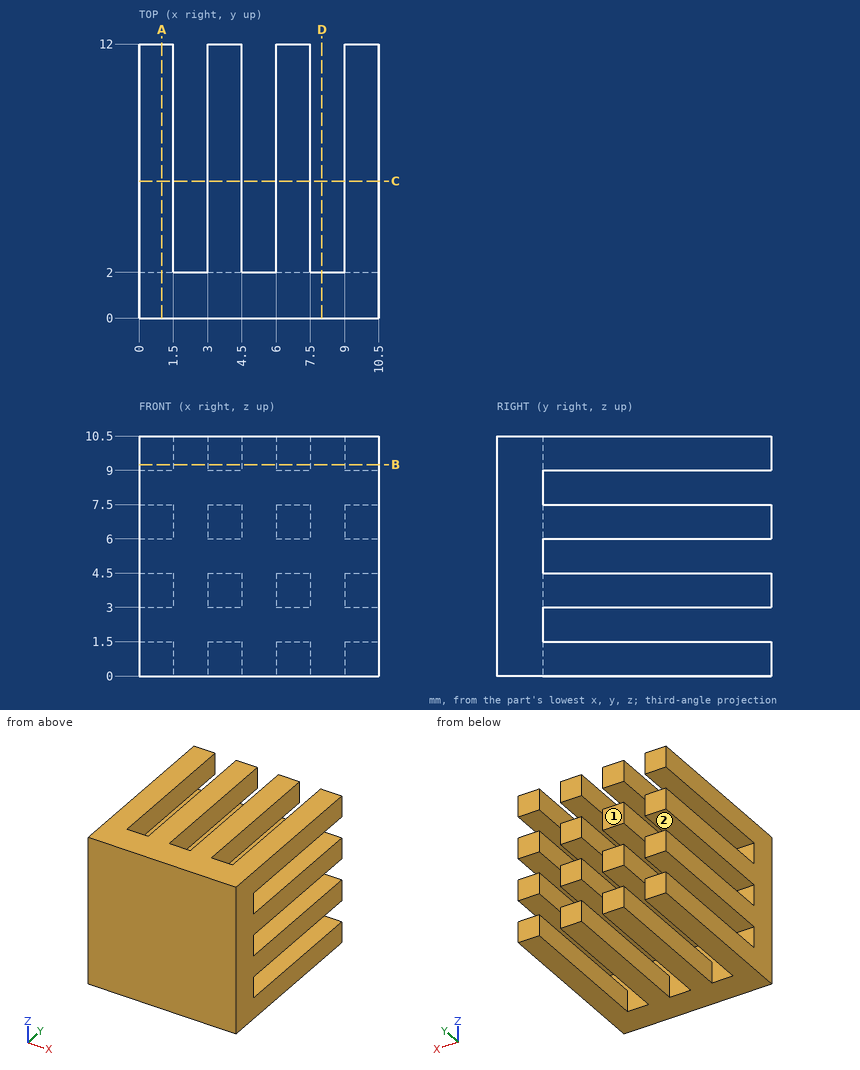
Can you work these out from the drawing? Everything is in mm from the part's minimum corner. A direction names the side the tool comes from. Round coordinates to 2 decimals unless told otherwise and drop trailing zeros. Order: outer loops, then holes, each group sorted by start corner. A loop starts at its lowest first (then second) coordinate and runs counter-clockwise, first axis right, second up. Notation, with made-up numbers: (66.5, 17) -> (109.5, 17) arc R7 ccw to (109.5, 27) -> close; hole circle Ø2 at (28, 60.25). An arc over 180 degrees is marked (long way). Return JSON: item names as keys, results as strings. Group by question number.
1. If we section it at C-C, the plane y = 6: Count the separate pieces of the cut face and the enclosed holes in it, then the cut area to 3 significant figures.
2. I need wall thicknesses on line 1 (Z direction, x = 1.25, y = 4.5); line 2 (Y direction, x = 5.25, z = 2.5). Which ranges of each line are inside material? Lowest first, please. Write a range as [from, to].
3. If we section it at A-A, the plane x = 1: Write out the boundary of the cut face in (y, z), then the cut area to 3 significant figures.
4. If we section it at B-B, the plane z = 9.25: Write out the boundary of the cut face in (x, y), then the cut area to 3 significant figures.
5. Which directions (+Z, -Z, +X, -X, +Y, -Y) give clear straight access to the entire face, cutting with the end or side of a thin tool? Please do the marked faces 1 and 2.
6. If we section it at D-D, the plane x = 8: Write out the boundary of the cut face in (y, z), then the cut area to 3 significant figures.
Output values:
{
 "1": {"separate pieces": "16", "enclosed holes": "0", "area": "36.0 mm²"},
 "2": {"line 1": "[0, 1.5], [3, 4.5], [6, 7.5], [9, 10.5]", "line 2": "[0, 2]"},
 "3": {"outline": "(0, 0) -> (12, 0) -> (12, 1.5) -> (2, 1.5) -> (2, 3) -> (12, 3) -> (12, 4.5) -> (2, 4.5) -> (2, 6) -> (12, 6) -> (12, 7.5) -> (2, 7.5) -> (2, 9) -> (12, 9) -> (12, 10.5) -> (0, 10.5) -> close", "area": "81.0 mm²"},
 "4": {"outline": "(0, 0) -> (10.5, 0) -> (10.5, 12) -> (9, 12) -> (9, 2) -> (7.5, 2) -> (7.5, 12) -> (6, 12) -> (6, 2) -> (4.5, 2) -> (4.5, 12) -> (3, 12) -> (3, 2) -> (1.5, 2) -> (1.5, 12) -> (0, 12) -> close", "area": "81.0 mm²"},
 "5": {"face 1": "+Z, -Z, +X, -X, +Y", "face 2": "+X, -X, +Y"},
 "6": {"outline": "(0, 0) -> (2, 0) -> (2, 10.5) -> (0, 10.5) -> close", "area": "21.0 mm²"}
}
